```python
from build123d import *

# Parameters (mm, degrees)
ESBO_O3_W                = 16
ESBO_O3_H                = 16
RESSALTO_EXTRUS_O1_DEPTH = 12
ESBO_O4_R                = 3
RESSALTO_EXTRUS_O2_DEPTH = 5
RESSALTO_EXTRUS_O2_TAPER = 26
RESSALTO_EXTRUS_O3_DEPTH = 12
FILETE1_R                = 2


with BuildPart() as part:
    # Esboço1 → Revolução1 (revolve)
    with BuildSketch(Plane.XY):
        Polygon((0, 51.659238703), (0, 1.659238703), (2, 1.659238703), (2, 2.659238703), (12.35, 2.659238703), (12.35, 3.659238703), (4, 3.659238703), (4, 6.103683147), (12.35, 6.103683147), (12.35, 7.103683147), (4, 7.103683147), (4, 9.548127592), (12.35, 9.548127592), (12.35, 10.548127592), (4, 10.548127592), (4, 12.992572036), (12.35, 12.992572036), (12.35, 13.992572036), (4, 13.992572036), (4, 16.437016481), (12.35, 16.437016481), (12.35, 17.437016481), (4, 17.437016481), (4, 19.881460925), (12.35, 19.881460925), (12.35, 20.881460925), (4, 20.881460925), (4, 23.32590537), (12.35, 23.32590537), (12.35, 24.32590537), (4, 24.32590537), (4, 26.770349814), (12.35, 26.770349814), (12.35, 27.770349814), (4, 27.770349814), (4, 30.214794259), (12.35, 30.214794259), (12.35, 31.214794259), (4, 31.214794259), (4, 33.659238703), (12.35, 33.659238703), (12.35, 34.659238703), (4, 34.659238703), (4, 39.959238703), (8, 39.959238703), (8, 42.659238703), (5.5, 42.659238703), (5.5, 48.159238703), (8, 48.159238703), (8, 51.659238703), align=None)
    revolve(axis=Axis((0, 51.659238703, 0), (0, -1, 0)))

    # Esboço3 → Ressalto-extrusão1 (add)
    with BuildSketch(Plane.XZ.offset(-1.659238703)):
        with Locations((0, 4)):
            Rectangle(ESBO_O3_W, ESBO_O3_H)
    extrude(amount=RESSALTO_EXTRUS_O1_DEPTH)

    # Esboço4 → Ressalto-extrusão2 (add)
    with BuildSketch(Plane.XZ.offset(10.340761297)):
        Circle(ESBO_O4_R)
    extrude(amount=RESSALTO_EXTRUS_O2_DEPTH, taper=RESSALTO_EXTRUS_O2_TAPER)

    # Esboço5 → Ressalto-extrusão3 (add)
    with BuildSketch(Plane(origin=(0, 51.659238703, 0), x_dir=(1, 0, 0), z_dir=(0, 1, 0))):
        Polygon((0, -6.92820323), (6, -3.464101615), (6, 3.464101615), (0, 6.92820323), (-6, 3.464101615), (-6, -3.464101615), align=None)
    extrude(amount=RESSALTO_EXTRUS_O3_DEPTH)

    # Filete1
    filete1_edges = [part.edges().sort_by_distance(p)[0] for p in [
        (-3, 63.659238703, 5.196152423),
        (3, 63.659238703, 5.196152423),
        (6, 63.659238703, 0),
        (3, 63.659238703, -5.196152423),
        (-3, 63.659238703, -5.196152423),
        (-6, 63.659238703, 0),
    ]]
    fillet(filete1_edges, radius=FILETE1_R)


solid = part.part
```
Build history of the part. All positions in model axes, mm. A direction names the side the tool comes from. Give positions to 0.01 mm unless a question says otherwise; leave off trailing zeros. Loops run counter-clockwise (first coordinate to the right, second up) from the corner with the lowest first, then second, coordinate; pieces in that order, holes last.
1) Band-saw the part on D-D on y = 8. List the corners of the cut face in (x, z), then the cut area to 3 significant figures.
Values follow:
outline: circle Ø8 at (0, 0)
area: 50.3 mm2
2) Two-plate mould, pull along Y, no slides. Class faces 1 (the face through (3, 23.326, 3)), 2 (the face through (0, -10.341, 4)), 3 (the face through (5.43, 63.06, -0.05)): released by +Y, released by -Y, zero draft, split by the parting line, or undercut.
Values follow:
face 1: undercut
face 2: released by -Y
face 3: released by +Y
3) 3-axis set-ups, long thin cutter, end or side, ignore diameter. For faces 4 (the face through (-1.73, 49.93, -7.81)), 5 (the face through (-0.867, 8.343, -3.905)), 6 (the face through (8, -4, 4)): which of +Z, -Z, +X, -X, +Y, -Y reach the whole face in a straight line?
Values follow:
face 4: +Y
face 5: none
face 6: +Z, -Z, +X, -Y
4) Band-saw the part on B-B on x = -4.75. State how many separate pieces and enclosed holes the cut face has, then the cut area to 3 significant figures.
Values follow:
separate pieces: 12
enclosed holes: 0
area: 628 mm2
5) Drop flat-ended pins along their axis: P1, Ø6, axis at y = -6, z = 5.5, coming from the +X side; P2, Ø5, axis at x = -1.5, y = 8, coming from the +Z side; P3, Ø13, axis at x = -3, y = -6, coming from the +Z side; P4, Ø3, axis at x = 8, y = 46.5, coming from the -Z side. Give the stop position or say it passes through.
Values follow:
P1: stops at x = 8
P2: stops at z = 12.35
P3: stops at z = 12
P4: passes through
6) Band-saw the part on A-A on y = 54.5. List the corners of the cut face in (x, z).
Values follow:
outline: (-6, -3.46) - (0, -6.93) - (6, -3.46) - (6, 3.46) - (0, 6.93) - (-6, 3.46) - close
7) Probe line 1 along Z through (x, y) = (6.25, -3); line 2 along X through (y, z) = (-6.5, -2.25); line 3 along X through (y, z) = (57.5, 0). List the from-to ranges inside material, lowest first.
Values follow:
line 1: z = -4 to 12
line 2: x = -8 to 8
line 3: x = -6 to 6
